The model under review builds one solid part; all positions refer to its coordinate system, in mm. Face numbers are marked on the shaded views. Round coordinates to 2 decimals unless told otherwise and drop trailing zeros. Loops run counter-clockwise (first coordinate to the right, second up) from the corner with the lowest first, then second, coordinate; pieces in that order, holes last. Notation, with made-up numbers: (14, -31.75) -> (47, -31.75) arc R21 ccw to (47, -26.75) -> close; hole circle Ø8 at (84.5, -31). An arc over 180 degrees is marked (long way). Use a Markdown table: item, result. Add a question column.
1) Wall thickness on probe 1 along Z at (x, y) = (1.8, 0); probe 2 along Z at (x, y) = (1.85, -0.5); probe 3 along Y at (x, z) = (1.9, -1): over which ranges is each line inside the solid? List them lowest first.
2) Insertion check: pin 1 (2 mm diameter, centred on y = 0, z = 0, fed in from -X). The pin has a flat end and moves straight along its axis. Give the tip position at first contact, or say it passes through.
3) Mouldability with a two-part tool opening along Z and no side actions: class the marked faces 1, 2 and 3 as released by +Z, released by -Z, zero draft, split by the parting line, or undercut.
4) Consider section A-A on x = 1.7. Give the boundary of the cut face in (y, z).
Autodesk Inventor part; units mm, degrees
ref_plane "Work Plane1" through (-5.9878, 0, 0) normal (0, -0.8660254, -0.5) x (1, 0, 0)
ref_plane "YZ Plane" through (0, 0, 0) normal (1, 0, 0) x (0, 1, 0)
ref_plane "XZ Plane" through (0, 0, 0) normal (0, 1, 0) x (-1, 0, 0)
sketch "Esquisse1" plane through (0, 0, 0) normal (1, 0, 0) x (0, 1, 0)
  line L0 (-3.1754, 0) -> (-1.5877, 2.75)
  line L1 (-1.5877, 2.75) -> (1.5877, 2.75)
  line L2 (1.5877, 2.75) -> (3.1754, 0)
  line L3 (3.1754, 0) -> (1.5877, -2.75)
  line L4 (1.5877, -2.75) -> (-1.5877, -2.75)
  line L5 (-1.5877, -2.75) -> (-3.1754, 0)
  point P0 (0, 0)
  point P1 (0, 0)
  dimension "d0" = 6.3509
extrude "Corps" add sketch "Esquisse1" along normal blind 2.9
sketch "Esquisse2" plane through (0, 0, 0) normal (0, 0, 1) x (1, 0, 0)
  line L0 (0, 1.5877) -> (0, 3.1754)
  line L1 (0, 3.1754) -> (2.9, 3.1754)
  line L2 (2.9, 1.5877) -> (2.9, 3.1754)
  line L3 (-0.58, 0) -> (3.48, 0)
  line L4 (0.2456, 3.1754) -> (0, 2.75)
  line L5 (2.6544, 3.1754) -> (2.9, 2.75)
  dimension "d3" = 30
  dimension "d4" = 30
  dimension "d5" = 5.5
  dimension "d6" = 5.5
revolve "Chanfrein1" cut sketch "Esquisse2" angle 360 about axis through (-10, 0, 0) along (1, 0, 0)
sketch "Esquisse3" plane through (2.9, 0, 0) normal (1, 0, 0) x (0, 0, -1)
  arc A0 (-1.375, -2.3816) -> (1.375, -2.3816) centre (0, 0) ccw
hole "Filetage" at (2.9, 0, 0) direction (-1, 0, 0) diameter 2.459 end through all
chamfer "Chanfrein2" distance 0.2706 angle 30 1 edges at (2.9, 0, 1.2295) measured on face at (2.9, -2.2301, -0.0494)
chamfer "Chanfrein3" distance 0.2706 angle 30 1 edges at (0, 0, 1.2295) measured on face at (0, -2.2301, -0.0494)
ref_plane "Work Plane1" through (-5.9878, 0, 0) normal (0, -0.8660254, -0.5) x (1, 0, 0)
equation "\"d0\" = 1.1547 * SW"
equation "\"d1\" = KOH"
equation "\"d3\" = ANG1"
equation "\"d4\" = ANG2"
equation "\"d5\" = SW0"
equation "\"d6\" = SW01"
equation "\"d8\" = -0.5 * GD1 + 0.5 * NND"
equation "\"d40\" = -0.5 * GD1 + 0.5 * NND"
equation "\"d10\" = -0.5 * GD1 + 0.5 * NND"
equation "\"d41\" = -0.5 * GD1 + 0.5 * NND"
equation "\"ANG1\" = 30deg"
equation "\"ANG2\" = 30deg"
equation "\"NND\" = 3"
equation "\"KOH\" = 2.9"
equation "\"SW\" = 5.5"
equation "\"SW0\" = SW"
equation "\"SW01\" = SW"
equation "\"GUL\" = 0.541266 * PTC"
equation "\"THREADDIA\" = 3"
equation "\"TOA\" = 30deg"
equation "\"PTC\" = 0.5"
equation "\"E0\" = 1.155 * SW"
equation "\"GAL\" = 0.541266 * PTC"
equation "\"SD2\" = 0"
equation "\"WFT\" = 0"
properties part number "ANSI B18.2.4.2M - M3 x 0,5" material "Acier, doux"
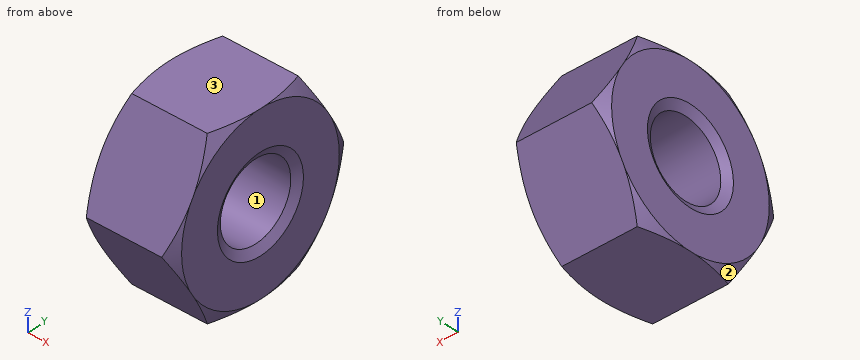
Result set:
| question | item | result |
|---|---|---|
| 1 | probe 1 | -2.75 to -1.23, 1.23 to 2.75 |
| 1 | probe 2 | -2.75 to -1.12, 1.12 to 2.75 |
| 1 | probe 3 | -2.6 to -0.72, 0.72 to 2.6 |
| 2 | pin 1 | through |
| 3 | face 1 | undercut |
| 3 | face 2 | released by -Z |
| 3 | face 3 | released by +Z |
| 4 | outline | (-3.18, 0) -> (-1.59, -2.75) -> (1.59, -2.75) -> (3.18, 0) -> (1.59, 2.75) -> (-1.59, 2.75) -> close; hole circle Ø2.46 at (0, 0) |
